Autodesk Inventor part; units mm, degrees
ref_plane "YZ Plane" through (0, 0, 0) normal (1, 0, 0) x (0, 1, 0)
ref_plane "XZ Plane" through (0, 0, 0) normal (0, 1, 0) x (-1, 0, 0)
ref_plane "XY Plane" through (0, 0, 0) normal (0, 0, 1) x (1, 0, 0)
sketch "Skizze1" plane through (0, 0, 0) normal (0, 1, 0) x (-1, 0, 0)
  line L0 (0, 0) -> (63, 0)
  line L1 (63, 0) -> (63, 145)
  line L2 (63, 145) -> (0, 145)
  line L3 (0, 145) -> (0, 0)
  line L4 (63, 0) -> (67, 0)
  line L5 (63, 123.7495) -> (63, 0)
  line L6 (0, 0) -> (-4, 0)
  line L7 (0, 125) -> (0, 0)
  line L8 (63, 0) -> (66.5, 0)
  line L9 (66.5, 0) -> (66.5, 145)
  line L10 (66.5, 145) -> (63, 145)
  line L11 (63, 145) -> (63, 0)
  line L12 (66.5, 145) -> (65, 145)
  line L13 (65, 145) -> (65, 0)
  line L14 (65, 0) -> (66.5, 0)
  line L15 (66.5, 0) -> (66.5, 145)
  line L16 (0, 0) -> (-3.5, 0)
  line L17 (-3.5, 0) -> (-3.5, 145)
  line L18 (-3.5, 145) -> (0, 145)
  line L19 (0, 145) -> (0, 0)
  line L20 (-3.5, 0) -> (-2, 0)
  line L21 (-2, 0) -> (-2, 145)
  line L22 (-2, 145) -> (-3.5, 145)
  line L23 (-3.5, 145) -> (-3.5, 0)
  line L24 (66.5, 145) -> (-3.5, 145)
  line L25 (-3.5, 145) -> (-3.5, 146.5)
  line L26 (-3.5, 146.5) -> (66.5, 146.5)
  line L27 (66.5, 146.5) -> (66.5, 145)
  line L28 (41.5, 145) -> (21.5, 145)
  line L29 (21.5, 145) -> (21.5, 146.5)
  line L30 (21.5, 146.5) -> (41.5, 146.5)
  line L31 (41.5, 146.5) -> (41.5, 145)
  point P0 (65, 0)
  point P1 (0, 145)
  point P2 (-2, 0)
  point P3 (-3.5, 0)
  dimension "d0" = 63
  dimension "d1" = 145
  dimension "d5" = 1.5
  dimension "d6" = 3.5
  dimension "d7" = 3.5
  dimension "d8" = 1.5
  dimension "d9" = 1.5
  dimension "d29" = 0
  dimension "d31" = 0
  dimension "d32" = 0
  dimension "d33" = 20
  dimension "d34" = 25
  dimension "d35" = 25
extrude "Extrusion1" add sketch "Skizze1" along normal blind 1.5 contours L3 L2 L1 L0 | L6 L21 L18 L3 | L1 L10 L13 L4
extrude "Extrusion2" add sketch "Skizze1" along normal blind 4 contours L6 L17 L18 L21 | L13 L10 L9 L4
sketch "Skizze2" plane through (0, 4, 0) normal (0, 1, 0) x (1, 0, 0)
  line L0 (-66.5, -145) -> (3.5, -145)
  line L1 (2, 0) -> (-65, 0)
  line L2 (3.5, -145) -> (0.5, -145)
  line L3 (0.5, -145) -> (0.5, 0)
  line L4 (0.5, 0) -> (3.5, 0)
  line L5 (3.5, 0) -> (3.5, -145)
  point P0 (0, 0)
  point P1 (-63, -125)
  point P2 (2, 0)
  point P3 (0.5, -144.0977)
  dimension "d14" = 3
extrude "Extrusion3" add sketch "Skizze2" along normal blind 1.5
sketch "Skizze3" plane through (0, 4, 0) normal (0, 1, 0) x (1, 0, 0)
  line L0 (-66.5, 0) -> (-66.5, -145)
  line L1 (-66.5, 0) -> (-63, 0)
  line L2 (-63, 0) -> (-63, -125.035)
  line L3 (-66.5, -125.035) -> (-66.5, 0)
  line L4 (-63, -125.035) -> (-63, -145)
  line L5 (-63, -145) -> (-66.5, -145)
  point P0 (0, 0)
  point P1 (-66.5, -125.035)
  dimension "d17" = 3.5
extrude "Extrusion4" add sketch "Skizze3" along normal blind 1.5
extrude "Extrusion5" add sketch "Skizze1" along normal blind 5.5 contours L18 L25 L26 L29 L2 | L2 L31 L26 L27 L10 | L29 L26 L31 L2
sketch "Skizze4" plane through (3.5, 0, 0) normal (0, 0, -1) x (-1, 0, 0)
  line L0 (1.5, 1.5) -> (68.5, 1.5)
  line L1 (0, 0) -> (70, 0)
  line L2 (1.5, 4) -> (3, 4)
  line L3 (0, 5.5) -> (3, 5.5)
  line L4 (0, 0) -> (0, 5.5)
  line L5 (3, 4) -> (3, 5.5)
  line L6 (1.5, 1.5) -> (1.5, 4)
  line L7 (68.5, 1.5) -> (68.5, 4)
  line L8 (66.5, 4) -> (66.5, 5.5)
  line L9 (70, 0) -> (70, 5.5)
  point P0 (3.5, 0)
  dimension "d22" = 1.5
  dimension "d23" = 2.5
  dimension "d24" = 1.5
  dimension "d25" = 3
  dimension "d26" = 1.5
  dimension "d27" = 67
  dimension "d28" = 63.5
  dimension "d30" = 70
extrude "Extrusion6" add sketch "Skizze1" along normal blind 20 contours L29 L26 L31 L2
properties part number "Deckel-Pumpe.v2"
Geometry check sheet. Reference: the model listing, model coordinates, mm. A direction names the side the tool comes from. Round coordinates to 2 decimals unless told otherwise and drop trailing zeros. Loops run counter-clockwise (first coordinate to the right, second up) from the corner with the lowest first, then second, coordinate; pieces in that order, holes last. Notation, with made-up numbers: (30, 52) - (58, 52) arc R19 cw to (58, 68) - close; hole circle Ø1 at (85.25, 31). An arc over 180 degrees is marked (long way). Use a Markdown table: item, result.
Q1. Draft check along Y on faces 1 (the flat face through (3.5, 3, 72)), 2 (the flat face through (-31, 0, 74)), 3 (the flat face through (2, 3, 71)). Enter one of: released by +Y, released by -Y, zero draft, split by the parting line, or undercut.
Solutions:
| item | result |
|---|---|
| face 1 | zero draft |
| face 2 | released by -Y |
| face 3 | undercut |
Q2. Cross-section at A-A on x = -51. Record the cut outline in (y, z), plus the area to 3 significant figures.
Solutions:
| item | result |
|---|---|
| outline | (0, 0) - (1.5, 0) - (1.5, 145) - (5.5, 145) - (5.5, 146.5) - (0, 146.5) - close |
| area | 226 mm2 |
Q3. Material ranges on line 1 (X direction, y = 5, z = 96); line 2 (Y direction, x = -13, z = 87); line 3 (Z direction, x = -37, y = 9.25), recorded low to high.
Solutions:
| item | result |
|---|---|
| line 1 | x = -66.5 to -63, 0.5 to 3.5 |
| line 2 | y = 0 to 1.5 |
| line 3 | z = 145 to 146.5 |
Q4. Cross-section at B-B on z = 49. Record the cut outline in (x, y).
Solutions:
| item | result |
|---|---|
| outline | (-66.5, 0) - (3.5, 0) - (3.5, 5.5) - (0.5, 5.5) - (0.5, 4) - (2, 4) - (2, 1.5) - (-65, 1.5) - (-65, 4) - (-63, 4) - (-63, 5.5) - (-66.5, 5.5) - close |
Q5. Access from +Z, -Z, +X, -X, +Y, -Y to the whole of each face (thin tool, end or side, straight path). Record for faces 4 (the flat face through (-65, 3, 74)), 5 (the flat face through (-32, 1, 0)).
Solutions:
| item | result |
|---|---|
| face 4 | -Z |
| face 5 | -Z, +X, -X, +Y, -Y |
Q6. Go/stop test with flat-tipped pins: P1, Ø20, axis at x = -7, z = 56, coming from the +Y side; P2, Ø1, axis at x = -14.5, y = 5, coming from the -Z side; P3, Ø7.5, axis at x = -54.5, z = 105, coming from the +Y side. Record where each tip stops, or that it passes through.
Solutions:
| item | result |
|---|---|
| P1 | stops at y = 5.5 |
| P2 | stops at z = 145 |
| P3 | stops at y = 1.5 |
Q7. Cross-section at C-C on y = 13.75. Record the cut outline in (x, z), plus the area to 3 significant figures.
Solutions:
| item | result |
|---|---|
| outline | (-41.5, 145) - (-21.5, 145) - (-21.5, 146.5) - (-41.5, 146.5) - close |
| area | 30.0 mm2 |
Q8. Cross-section at D-D on x = -29.5. Record the cut outline in (y, z), plus the area to 4 significant figures.
Solutions:
| item | result |
|---|---|
| outline | (0, 0) - (1.5, 0) - (1.5, 145) - (20, 145) - (20, 146.5) - (0, 146.5) - close |
| area | 247.5 mm2 |
